Design review of the part built by this model. Coordinates are the model's own, in mm. Coordinates: 2 decimals unless noted, no trailing zeros. Order: outer loops, then holes, each group sorted by start corner. A loop starts at its lowest first (then second) coordinate and runs counter-clockwise, first axis right, second up.
from build123d import *

# Parameters (mm, degrees)
SKETCH1_W           = 96
SKETCH1_H           = 113.24
BOSS_EXTRUDE1_DEPTH = 7
SKETCH2_R           = 1.59
CUT_EXTRUDE1_DEPTH  = 10
SKETCH4_R           = 2
CUT_EXTRUDE3_DEPTH  = 197.849722269


with BuildPart() as part:
    # Sketch1 → Boss-Extrude1 (new body)
    with BuildSketch(Plane.XY):
        with Locations((-112.864898463, 42.367863248)):
            Rectangle(SKETCH1_W, SKETCH1_H)
    extrude(amount=BOSS_EXTRUDE1_DEPTH)

    # Sketch2 → Cut-Extrude1 (cut)
    with BuildSketch(Plane.XY.offset(7)):
        with Locations((-152.234898463, 82.899456576)):
            Circle(SKETCH2_R)
        with Locations((-72.264898463, 82.899456576)):
            Circle(SKETCH2_R)
        with Locations((-149.694898463, -2.792907728)):
            Circle(SKETCH2_R)
        with Locations((-76.034898463, -2.792907728)):
            Circle(SKETCH2_R)
    extrude(amount=-CUT_EXTRUDE1_DEPTH, mode=Mode.SUBTRACT)

    # Sketch4 → Cut-Extrude3 (cut, through all)
    with BuildSketch(Plane(origin=(0, 98.987863248, 0), x_dir=(1, 0, 0), z_dir=(0, 1, 0))):
        with Locations(Location((-67.864898463, -3.5, 0), (0, 0, 270))):
            Circle(SKETCH4_R)
        with Locations(Location((-157.864898463, -3.5, 0), (0, 0, 270))):
            Circle(SKETCH4_R)
    extrude(amount=-CUT_EXTRUDE3_DEPTH, mode=Mode.SUBTRACT)


solid = part.part
1. To check wall thickness, follow line 1 (X direction, y = 72.5, z = 3.75); line 2 (X direction, y = 34.5, z = 3.5). State the ranges of each line that lie inside material, in increasing order.
2. Add section B-B (y = 90.5). Give the boundary of the cut face in (x, z).
3. Add section A-A (z = 3.5). Give the boundary of the cut face in (x, y).
4. Insertion check: pin 1 (3 mm diameter, centred on x = -67.86, z = 3.5, fed in from -Y). The pin has a flat end and moves straight along its axis. Give the tip position at first contact, or say it passes through.
5. Mouldability with a two-part tool opening along Y and no side actions: class faces 1 (the flat face through (-64.865, 42, 3)), 2 (the cylindrical face through (-151.283, -2.723, 3.549)), 3 (the flat face through (-114, 98.988, 3)) as pulls with the +Y half, pulls with the -Y half, needs draft (parallel to the pull), parting line crosses it, or undercut.
Solution:
1. line 1: x = -160.86 to -159.85, -155.88 to -69.85, -65.88 to -64.86
1. line 2: x = -160.86 to -159.86, -155.86 to -69.86, -65.86 to -64.86
2. outline: (-160.86, 0) - (-64.86, 0) - (-64.86, 7) - (-160.86, 7) - close; hole circle Ø4 at (-157.86, 3.5); hole circle Ø4 at (-67.86, 3.5)
3. outline: (-160.86, -14.25) - (-159.86, -14.25) - (-159.86, 98.99) - (-160.86, 98.99) - close; (-155.86, -14.25) - (-69.86, -14.25) - (-69.86, 98.99) - (-155.86, 98.99) - close; (-65.86, -14.25) - (-64.86, -14.25) - (-64.86, 98.99) - (-65.86, 98.99) - close; hole circle Ø3.18 at (-152.23, 82.9); hole circle Ø3.18 at (-149.69, -2.79); hole circle Ø3.18 at (-76.03, -2.79); hole circle Ø3.18 at (-72.26, 82.9)
4. pin 1: passes through
5. face 1: needs draft
5. face 2: undercut
5. face 3: pulls with the +Y half
